Here's the drawing with two shaded views (mm, measured from the low corner). I have some questions. A direction names the side the tool comes from. Round coordinates to 2 decimals unless told otherwise and drop trailing zeros. Order: outer loops, then holes, each group sorted by start corner. A loop starts at its lowest first (then second) coordinate and runs counter-clockwise, first axis right, second up. Notation, with made-up numbers: (18.25, 13.25) - (75.25, 13.25) arc R26 ccw to (75.25, 27.25) - close; hole circle Ø10 at (-18.5, 64). An arc over 180 degrees is marked (long way). Return JSON: item names as keys, results as strings. Group by question number.
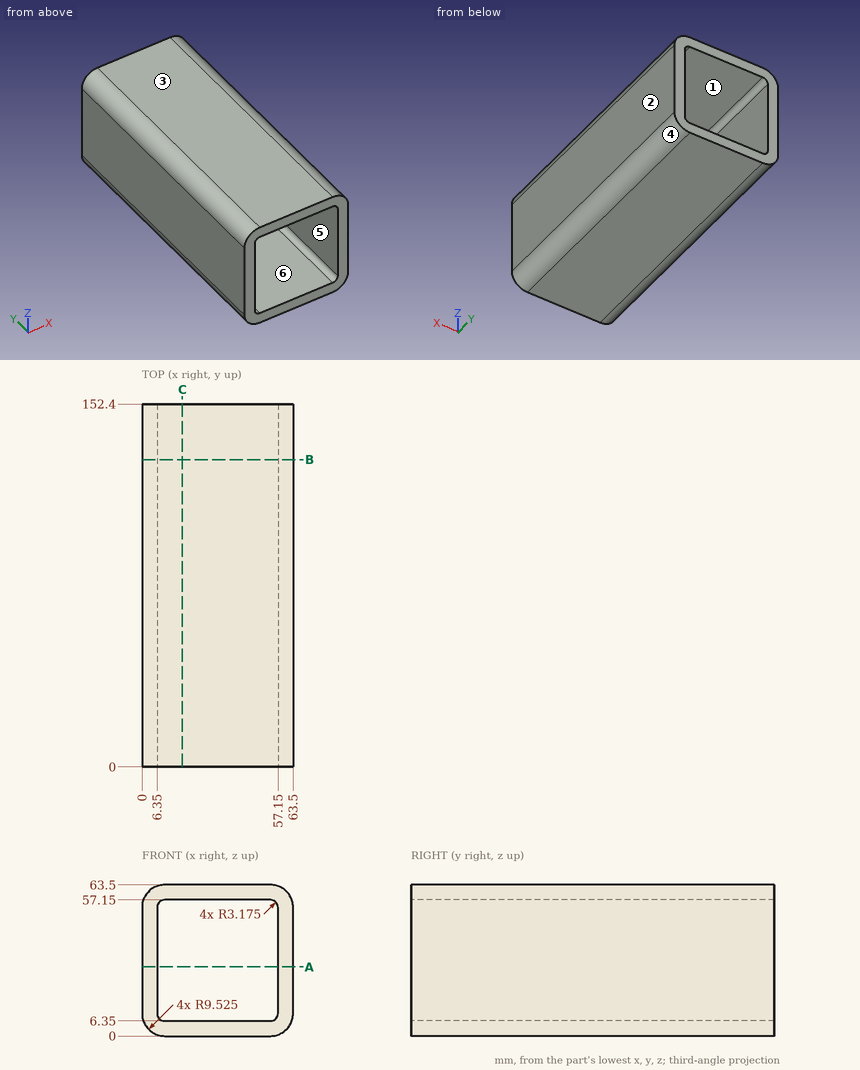
1) If I drill on line 1 along X through (y, z) = (18, 37), over which ranges is the centre line in solid material (lowest first)? Write a range as from..to.
2) I want a section at A-A, the plane z = 29. List the corners of the cut face in (x, y) for me.
3) I want a section at C-C, the plane x = 17. List the corners of the cut face in (y, z) for me.
4) We'd pull the mould along X, two halves only. Please class the marked faces 3, 4, 5 and 6: +X half, -X half, draft (parallel to the pull), parting line (faces both ways), or undercut.
5) For the marked faces 1 and 2, which set-ups out of +Z, -Z, +X, -X, +Y, -Y let a thin tool reach every point of the face, with its end or its side?
6) I want a section at B-B, the plane y = 129. List the corners of the cut face in (x, z) for me (3 decimals), plus the area to 3 significant figures.
Outcome:
{
 "1": {"line 1": "0..6.35, 57.15..63.5"},
 "2": {"outline": "(0, 0) - (6.35, 0) - (6.35, 152.4) - (0, 152.4) - close; (57.15, 0) - (63.5, 0) - (63.5, 152.4) - (57.15, 152.4) - close"},
 "3": {"outline": "(0, 0) - (152.4, 0) - (152.4, 6.35) - (0, 6.35) - close; (0, 57.15) - (152.4, 57.15) - (152.4, 63.5) - (0, 63.5) - close"},
 "4": {"face 3": "draft", "face 4": "+X half", "face 5": "undercut", "face 6": "undercut"},
 "5": {"face 1": "+Y, -Y", "face 2": "+Z, -Z, +X, +Y, -Y"},
 "6": {"outline": "(0, 9.525) arc R9.525 ccw to (9.525, 0) - (53.975, 0) arc R9.525 ccw to (63.5, 9.525) - (63.5, 53.975) arc R9.525 ccw to (53.975, 63.5) - (9.525, 63.5) arc R9.525 ccw to (0, 53.975) - close; hole (6.35, 9.525) arc R3.175 ccw to (9.525, 6.35) - (53.975, 6.35) arc R3.175 ccw to (57.15, 9.525) - (57.15, 53.975) arc R3.175 ccw to (53.975, 57.15) - (9.525, 57.15) arc R3.175 ccw to (6.35, 53.975) - close", "area": "1,380 mm^2"}
}
